The listing builds one solid part. Answer for the finished solid, in the listing's coordinates (mm). Give positions to 0.01 mm unless a question says otherwise; leave off trailing zeros. Order: outer loops, then holes, each group sorted by start corner. A loop starts at its lowest first (then second) coordinate and runs counter-clockwise, first axis right, second up. Notation, with made-up numbers: (84, 53) - (113, 53) arc R20 ccw to (113, 70) - close; hole circle Ø2 at (64, -16.75). An arc over 180 degrees is marked (long way). Use a Markdown table: item, result. Add a question column.
1) Straight lines are drawn through the part: line 1 (Z direction, x = -7.25, y = 364.5); line 2 (X direction, y = 189, z = -15); line 3 (Y direction, x = -2.75, z = -14). For each, find the intervals that lie inside material, in ascending order.
2) Find section A-A, the plane x = -9.75. Determine the outline of the cut face in (y, z).
3) A flat-ended cylindrical pin translates along its axis: pin 1 (1 mm diameter, centred on x = -8.5, z = -14.5, fed in from +Y). Find the tip coordinate at first contact, or state that the pin passes through.
4) Find section B-B, the plane z = -7.75. Determine the outline of the cut face in (x, y), plus the area to 3 significant figures.
5) Find section C-C, the plane y = 429. Determine the outline of the cut face in (x, z).
from build123d import *

# Parameters (mm, degrees)
SKETCH1_W           = 13
SKETCH1_H           = 13
BOSS_EXTRUDE1_DEPTH = 558.8
SHELL1_T            = -1.5875
FILLET1_R           = 1.524
FILLET2_R           = 1.524


with BuildPart() as part:
    # Sketch1 → Boss-Extrude1 (new body)
    with BuildSketch(Plane(origin=(0, 0, 0), x_dir=(1, 0, 0), z_dir=(0, 1, 0))):
        with Locations((-9.0448, 10.3402)):
            Rectangle(SKETCH1_W, SKETCH1_H)
    extrude(amount=BOSS_EXTRUDE1_DEPTH)

    # Shell1
    shell1_openings = [part.faces().sort_by_distance(p)[0] for p in [
        (-9.0448, 558.8, -10.3402),
        (-9.0448, 0, -10.3402),
    ]]
    offset(amount=SHELL1_T, openings=shell1_openings, kind=Kind.INTERSECTION)

    # Fillet1
    fillet1_edges = [part.edges().sort_by_distance(p)[0] for p in [
        (-13.9573, 0, -10.3402),
        (-9.0448, 0, -5.4277),
        (-4.1323, 0, -10.3402),
        (-9.0448, 0, -15.2527),
    ]]
    fillet(fillet1_edges, radius=FILLET1_R)

    # Fillet2
    fillet2_edges = [part.edges().sort_by_distance(p)[0] for p in [
        (-13.9573, 558.8, -10.3402),
        (-9.0448, 558.8, -5.4277),
        (-4.1323, 558.8, -10.3402),
        (-9.0448, 558.8, -15.2527),
    ]]
    fillet(fillet2_edges, radius=FILLET2_R)


solid = part.part
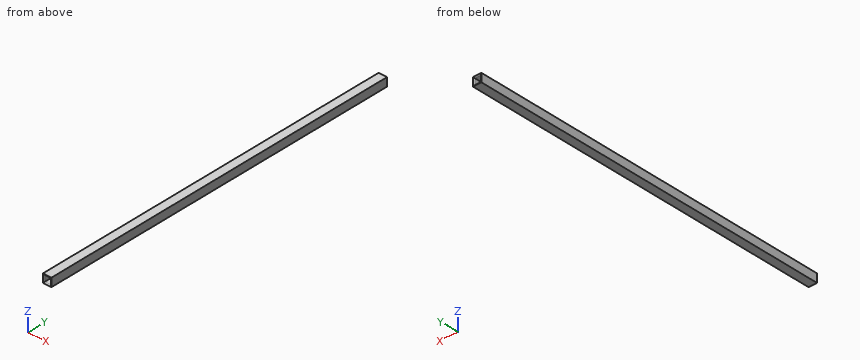
The answers:
| question | item | result |
|---|---|---|
| 1 | line 1 | -16.84 to -15.25, -5.43 to -3.84 |
| 1 | line 2 | -15.54 to -13.96, -4.13 to -2.54 |
| 1 | line 3 | 0.01 to 558.79 |
| 2 | outline | (0, -16.84) - (558.8, -16.84) - (558.8, -16.78) arc R1.52 ccw to (557.28, -15.25) - (1.52, -15.25) arc R1.52 ccw to (0, -16.78) - close; (0, -3.9) arc R1.52 ccw to (1.52, -5.43) - (557.28, -5.43) arc R1.52 ccw to (558.8, -3.9) - (558.8, -3.84) - (0, -3.84) - close |
| 3 | pin 1 | through |
| 4 | outline | (-15.54, 0) - (-15.48, 0) arc R1.52 ccw to (-13.96, 1.52) - (-13.96, 557.28) arc R1.52 ccw to (-15.48, 558.8) - (-15.54, 558.8) - close; (-4.13, 1.52) arc R1.52 ccw to (-2.61, 0) - (-2.54, 0) - (-2.54, 558.8) - (-2.61, 558.8) arc R1.52 ccw to (-4.13, 557.28) - close |
| 4 | area | 1,770 mm2 |
| 5 | outline | (-15.54, -16.84) - (-2.54, -16.84) - (-2.54, -3.84) - (-15.54, -3.84) - close; hole (-13.96, -15.25) - (-4.13, -15.25) - (-4.13, -5.43) - (-13.96, -5.43) - close |
